Geometry: final body of the model. Coordinates: model frame, mm. A direction names the side the tool comes from. Give positions to 0.01 mm unless a question says otherwise; leave off trailing zeros. Loops run counter-clockwise (first coordinate to the right, second up) from the corner with the lowest first, then second, coordinate; pieces in that order, holes last.
```python
from build123d import *

# Parameters (mm, degrees)
RESSALTO_EXTRUS_O1_DEPTH   = 15
ESBO_O2_R                  = 2.25
CORTE_EXTRUS_O1_DEPTH      = 41.215045787
CORTE_EXTRUS_O2_DEPTH      = 46.367938746
CORTE_EXTRUS_O2_DEPTH_BACK = 46.367938746
ESBO_O3_R                  = 2.25
RESSALTO_EXTRUS_O2_DEPTH   = 8
CORTE_EXTRUS_O3_DEPTH      = 4
CORTE_EXTRUS_O4_REACH      = 69.72
CORTE_EXTRUS_O4_END_RADIUS = 2.75
ESBO_O6_R                  = 1.6
CORTE_EXTRUS_O5_DEPTH      = 3
ESBO_O8_R                  = 12.5
CORTE_EXTRUS_O6_DEPTH      = 15
CORTE_EXTRUS_O7_DEPTH      = 53.646110388
CORTE_EXTRUS_O7_DEPTH_BACK = 53.646110388
ESBO_O10_R                 = 5
CORTE_EXTRUS_O8_DEPTH      = 6
ESBO_O11_R                 = 5
CORTE_EXTRUS_O9_DEPTH      = 4


with BuildPart() as part:
    # Esboço1 → Ressalto-extrusão1 (new body)
    with BuildSketch(Plane.XY):
        Polygon((-28.499998137, 19.99999769), (-31.5, 16.99999769), (-31.5, -2.360471354), (-19.999999046, -9), (-3, -9), (0, -6), (0, 0), (-19.999999046, 0), (-19.999999046, 7.17), (-18.999999046, 7.17), (-18.999999046, 12.82999769), (-19.999999046, 12.82999769), (-19.999999046, 19.99999769), align=None)
    extrude(amount=RESSALTO_EXTRUS_O1_DEPTH)

    # Esboço2 → Corte-extrusão1 (cut, through all)
    with BuildSketch(Plane.ZY.offset(31.5)):
        with Locations((7.5, 9.99999769)):
            Circle(ESBO_O2_R)
    extrude(amount=-CORTE_EXTRUS_O1_DEPTH, mode=Mode.SUBTRACT)

    # Esboço3 → Corte-extrusão2 (cut, two sides: drawn at the far end of the back side and taken through both)
    with BuildSketch(Plane.XZ.offset(9).offset(-CORTE_EXTRUS_O2_DEPTH_BACK)):
        with Locations(Location((-9.999999046, 7.5, 0), (0, 0, 270))):
            Circle(ESBO_O3_R)
    extrude(amount=CORTE_EXTRUS_O2_DEPTH + CORTE_EXTRUS_O2_DEPTH_BACK, mode=Mode.SUBTRACT)

    # Esboço4 → Ressalto-extrusão2 (add)
    # profile 1 of 2: a face of its own
    with BuildSketch(Plane.XY.offset(15)):
        Polygon((-19.999999046, -9), (-31.5, -2.360471354), (-31.5, -35.360471354), (-19.999999046, -35.360471354), (0, -6), (-3, -9), align=None)
        with BuildLine():
            ThreePointArc((-22.25, -22.360471354), (-25, -25.110471354), (-27.75, -22.360471354))
            Line((-27.75, -22.360471354), (-27.75, -15.360471354))
            ThreePointArc((-27.75, -15.360471354), (-25, -12.610471354), (-22.25, -15.360471354))
            Line((-22.25, -15.360471354), (-22.25, -22.360471354))
        make_face(mode=Mode.SUBTRACT)
    # profile 2 of 2: a face of its own
    with BuildSketch(Plane.XY.offset(15)):
        Polygon((-31.5, 16.99999769), (-31.5, -2.360471354), (-19.999999046, -9), (-3, -9), (0, -6), (0, 0), (-19.999999046, 0), (-19.999999046, 7.17), (-18.999999046, 7.17), (-18.999999046, 12.82999769), (-19.999999046, 12.82999769), (-19.999999046, 19.99999769), (-28.499998137, 19.99999769), align=None)
    ressalto_extrus_o2 = extrude(amount=RESSALTO_EXTRUS_O2_DEPTH)

    # Espelhar1: Ressalto-extrusão2 across plane
    add(ressalto_extrus_o2.mirror(Plane.XY.offset(7.5)))

    # Esboço5 → Corte-extrusão3 (cut)
    with BuildSketch(Plane(origin=(0, 0, -8), x_dir=(-1, 0, 0), z_dir=(0, 0, -1))):
        Polygon((20.93, -17.9), (20.93, -24.710286949), (25, -27.060102545), (29.07, -24.710286949), (29.07, -17.9), (29.07, -13.010655758), (25, -10.660840163), (20.93, -13.010655758), align=None)
        with BuildLine():
            Line((22.25, -22.360471354), (22.25, -15.360471354))
            ThreePointArc((22.25, -15.360471354), (25, -12.610471354), (27.75, -15.360471354))
            Line((27.75, -15.360471354), (27.75, -22.360471354))
            ThreePointArc((27.75, -22.360471354), (25, -25.110471354), (22.25, -22.360471354))
        make_face(mode=Mode.SUBTRACT)
    extrude(amount=-CORTE_EXTRUS_O3_DEPTH, mode=Mode.SUBTRACT)

    # Corte-extrusão4: up to this cylinder (the profile starts outside it)
    corte_extrus_o4_end = Plane(origin=(-25, -22.360471354, 7.5), z_dir=(0, 0, -1)) * Cylinder(CORTE_EXTRUS_O4_END_RADIUS, 168.94, mode=Mode.PRIVATE)
    # Esboço6 → Corte-extrusão4 (cut, up to the surface)
    with BuildSketch(Plane.XZ.offset(35.360471354), mode=Mode.PRIVATE) as corte_extrus_o4_sk1:
        with Locations(Location((-25, 19, 0), (0, 0, 270))):
            Circle(ESBO_O6_R)
    corte_extrus_o4_tool1 = extrude(corte_extrus_o4_sk1.sketch, amount=-CORTE_EXTRUS_O4_REACH, mode=Mode.PRIVATE) - corte_extrus_o4_end
    add(corte_extrus_o4_tool1.solids().sort_by_distance((-25, -35.360471, 19))[0], mode=Mode.SUBTRACT)
    # Esboço6 → Corte-extrusão4 (cut, up to the surface)
    with BuildSketch(Plane.XZ.offset(35.360471354), mode=Mode.PRIVATE) as corte_extrus_o4_sk2:
        with Locations(Location((-25, -4, 0), (0, 0, 270))):
            Circle(ESBO_O6_R)
    corte_extrus_o4_tool2 = extrude(corte_extrus_o4_sk2.sketch, amount=-CORTE_EXTRUS_O4_REACH, mode=Mode.PRIVATE) - corte_extrus_o4_end
    add(corte_extrus_o4_tool2.solids().sort_by_distance((-25, -35.360471, -4))[0], mode=Mode.SUBTRACT)

    # Esboço7 → Corte-extrusão5 (cut)
    with BuildSketch(Plane(origin=(0, -32.360471354, 0), x_dir=(-1, 0, 0), z_dir=(0, -1, 0))):
        Polygon((26.674315781, -21.9), (33, -21.9), (33, -16.1), (26.674315781, -16.1), (23.325684219, -16.1), (21.651368439, -19), (23.325684219, -21.9), align=None)
        Polygon((26.674315781, 6.9), (23.325684219, 6.9), (21.651368439, 4), (23.325684219, 1.1), (26.674315781, 1.1), (33, 1.1), (33, 6.9), align=None)
    extrude(amount=-CORTE_EXTRUS_O5_DEPTH, mode=Mode.SUBTRACT)

    # Esboço8 → Corte-extrusão6 (cut)
    with BuildSketch(Plane.XY):
        with Locations((-25, -15.360471354)):
            Circle(ESBO_O8_R)
    extrude(amount=CORTE_EXTRUS_O6_DEPTH, mode=Mode.SUBTRACT)

    # Esboço9 → Corte-extrusão7 (cut, two sides: drawn at the far end of the back side and taken through both)
    with BuildSketch(Plane.ZY.offset(31.5).offset(-CORTE_EXTRUS_O7_DEPTH_BACK)):
        Polygon((-8, 0), (2.5, 19.99999769), (12.5, 19.99999769), (23, 0), (23, 29.458791051), (-8, 29.458791051), align=None)
    extrude(amount=CORTE_EXTRUS_O7_DEPTH + CORTE_EXTRUS_O7_DEPTH_BACK, mode=Mode.SUBTRACT)

    # Esboço10 → Corte-extrusão8 (cut)
    with BuildSketch(Plane.ZY.offset(31.5)):
        with Locations((7.5, 9.99999769)):
            Circle(ESBO_O10_R)
    extrude(amount=-CORTE_EXTRUS_O8_DEPTH, mode=Mode.SUBTRACT)

    # Esboço11 → Corte-extrusão9 (cut)
    with BuildSketch(Plane.XZ.offset(9)):
        with Locations((-9.999999046, 7.5)):
            Circle(ESBO_O11_R)
    extrude(amount=-CORTE_EXTRUS_O9_DEPTH, mode=Mode.SUBTRACT)


solid = part.part
```
Q1. Mould query, pull axis Z, two halves, no side actions, for faces 1 (the face through (-22.477, -30.881, 20.43)), 2 (the face through (-19, -14, 23)), 3 (the face through (-25.162, 9.86, -2.823)), 4 (the face through (-7.6, 0, 7.7)). Classes: +Z half, -Z half, draft (parallel to the pull), parting line (faces both ways), or undercut.
Q2. Section query C-C, the plane y = -24. Return loops of the section in (x, z), and give its area (3 significant figures).
Q3. Section query D-D, the plane x = -16. Return loops of the section in (y, z), and give its area (3 significant figures).
Q4. Section query B-B, the plane x = -10. Return loops of the section in (y, z).
Q5. Reachability of faces 5 (the face through (-22.94, -25.87, -6.03)), 6 (the face through (-28.54, 11.5, 12.27)), 7 (the face through (-22.25, -19, -2)) from +Z, -Z, +X, -X, +Y, -Y: full face, straight path, thin tool, end or side. Return the list, or none.
Q6. Section query A-A, the plane z = 7.5. State how many separate pieces and enclosed holes the cut face has, and give its area (3 significant figures).
Q7. Pin query (flat end, axial travel): pin 1 Ø4 at (y, z) = (-9, 6) entering from +X; pin 2 Ø7 at (y, z) = (10, 7.5) entering from -X; pin 3 Ø4.5 at (x, z) = (-25, -5) entering from +Y. Return the tip coordinate at first contact, or that it passes through.
Q8. Material intervals for probe 1 along Z at (x, y) = (-25, -25.7); probe 2 along Z at (x, y) = (-20, -30); probe 3 along Z at (x, y) = (-10, -7), sorted ascending.
Resolved:
1. face 1: undercut
1. face 2: +Z half
1. face 3: -Z half
1. face 4: draft
2. outline: (-31.5, -8) - (-29.07, -8) - (-29.07, -4) - (-27.21, -4) - (-27.21, 0) - (-31.5, 0) - close; (-31.5, 15) - (-27.21, 15) - (-27.21, 23) - (-31.5, 23) - close; (-22.79, -4) - (-20.93, -4) - (-20.93, -8) - (-12.26, -8) - (-12.26, 0) - (-22.79, 0) - close; (-22.79, 15) - (-12.26, 15) - (-12.26, 23) - (-22.79, 23) - close
2. area: 222 mm2
3. outline: (-29.49, -8) - (0, -8) - (0, 23) - (-29.49, 23) - (-29.49, 15) - (-6.69, 15) - (-6.69, 0) - (-29.49, 0) - close
3. area: 572 mm2
4. outline: (-20.68, -8) - (0, -8) - (0, 5.25) - (-5, 5.25) - (-5, 2.5) - (-9, 2.5) - (-9, 0) - (-20.68, 0) - close; (-20.68, 15) - (-9, 15) - (-9, 12.5) - (-5, 12.5) - (-5, 9.75) - (0, 9.75) - (0, 23) - (-20.68, 23) - close
5. face 5: -Z
5. face 6: -X
5. face 7: +Z, -Z
6. separate pieces: 3
6. enclosed holes: 0
6. area: 274 mm2
7. pin 1: stops at x = -1
7. pin 2: stops at x = -25.5
7. pin 3: stops at y = 10
8. probe 1: z = -2.4 to 0, 15 to 17.4, 20.6 to 23
8. probe 2: z = -8 to 0, 15 to 23
8. probe 3: z = -8 to 2.5, 12.5 to 23
